from build123d import *

# Parameters (mm, degrees)
CROQUIS1_W              = 195
CROQUIS1_H              = 38
CROQUIS1_R              = 1.625
SALIENTE_EXTRUIR1_DEPTH = 3
SALIENTE_EXTRUIR2_START = -20
SALIENTE_EXTRUIR2_DEPTH = 16.5
CROQUIS3_W              = 10.5
CROQUIS3_H              = 7
CORTAR_EXTRUIR1_DEPTH   = 31.243984
SALIENTE_EXTRUIR3_START = -20
SALIENTE_EXTRUIR3_DEPTH = 16.5
CROQUIS5_W              = 10.5
CROQUIS5_H              = 7
CORTAR_EXTRUIR2_DEPTH   = 31.243984
SALIENTE_EXTRUIR4_START = -120
SALIENTE_EXTRUIR4_DEPTH = 45
CROQUIS7_R              = 8.25
CORTAR_EXTRUIR3_DEPTH   = 31.243984
CROQUIS8_W              = 195
CROQUIS8_H              = 3
SALIENTE_EXTRUIR5_DEPTH = 5
CORTAR_EXTRUIR4_REACH   = 122
CROQUIS10_W             = 55.675323807
CROQUIS10_H             = 32.604384831
SALIENTE_EXTRUIR7_DEPTH = 3


with BuildPart() as part:
    # Croquis1 → Saliente-Extruir1 (new body)
    with BuildSketch(Plane.XY):
        with Locations((0, 19)):
            Rectangle(CROQUIS1_W, CROQUIS1_H)
        with Locations((91.125, 15)):
            Circle(CROQUIS1_R, mode=Mode.SUBTRACT)
        with Locations((-91.125, 15)):
            Circle(CROQUIS1_R, mode=Mode.SUBTRACT)
    extrude(amount=SALIENTE_EXTRUIR1_DEPTH)

    # Croquis2 → Saliente-Extruir2 (add)
    with BuildSketch(Plane(origin=(97.5, 0, 0), x_dir=(0, 0, -1), z_dir=(1, 0, 0)).offset(SALIENTE_EXTRUIR2_START)):
        Polygon((3.429565646, 3.677896428), (15.185426147, 13.753887502), (0, 31.471028189), (0, 0.738403157), align=None)
    extrude(amount=-SALIENTE_EXTRUIR2_DEPTH)

    # Croquis3 → Cortar-Extruir1 (cut, through all)
    with BuildSketch(Plane(origin=(0, 0.425684191, 0.364855478), x_dir=(1, 0, 0), z_dir=(0, -0.759271307, -0.650774217))):
        with Locations((69.25, -11.980533736)):
            Rectangle(CROQUIS3_W, CROQUIS3_H)
    extrude(amount=-CORTAR_EXTRUIR1_DEPTH, mode=Mode.SUBTRACT)

    # Croquis4 → Saliente-Extruir3 (add)
    with BuildSketch(Plane.ZY.offset(97.5).offset(SALIENTE_EXTRUIR3_START)):
        Polygon((0, 0.738403157), (-15.185426147, 13.753887502), (0, 31.471028189), align=None)
    extrude(amount=-SALIENTE_EXTRUIR3_DEPTH)

    # Croquis5 → Cortar-Extruir2 (cut, through all)
    with BuildSketch(Plane(origin=(0, 0.425684191, 0.364855478), x_dir=(1, 0, 0), z_dir=(0, -0.759271307, -0.650774217))):
        with Locations((-69.25, -11.980533736)):
            Rectangle(CROQUIS5_W, CROQUIS5_H)
    extrude(amount=-CORTAR_EXTRUIR2_DEPTH, mode=Mode.SUBTRACT)

    # Croquis6 → Saliente-Extruir4 (add)
    with BuildSketch(Plane(origin=(97.5, 0, 0), x_dir=(0, 0, -1), z_dir=(1, 0, 0)).offset(SALIENTE_EXTRUIR4_START)):
        Polygon((0, 0.738403157), (15.185426147, 13.753887502), (0, 31.471028189), align=None)
    extrude(amount=SALIENTE_EXTRUIR4_DEPTH)

    # Croquis7 → Cortar-Extruir3 (cut, through all)
    with BuildSketch(Plane(origin=(0, 0.425684191, 0.364855478), x_dir=(1, 0, 0), z_dir=(0, -0.759271307, -0.650774217))):
        with Locations((-12.92, -10.480533736)):
            Circle(CROQUIS7_R)
        with Locations((12.93, -10.480533736)):
            Circle(CROQUIS7_R)
    extrude(amount=-CORTAR_EXTRUIR3_DEPTH, mode=Mode.SUBTRACT)

    # Croquis8 → Saliente-Extruir5 (add)
    with BuildSketch(Plane.XZ):
        with Locations((0, 1.5)):
            Rectangle(CROQUIS8_W, CROQUIS8_H)
    extrude(amount=SALIENTE_EXTRUIR5_DEPTH)

    # Croquis9 → Cortar-Extruir4 (cut, up to next)
    with BuildSketch(Plane.ZY.offset(22.5), mode=Mode.PRIVATE) as cortar_extruir4_sk1:
        Polygon((0, 0.738403157), (-15.185426147, 13.753887502), (0, 31.471028189), align=None)
    cortar_extruir4_tool1 = extrude(cortar_extruir4_sk1.sketch, amount=-CORTAR_EXTRUIR4_REACH, mode=Mode.PRIVATE) & part.part
    add(cortar_extruir4_tool1.solids().sort_by_distance((-22.5, 15.321106, -5.061809))[0], mode=Mode.SUBTRACT)

    # Croquis10 → Saliente-Extruir7 (add)
    with BuildSketch(Plane.XY.offset(3)):
        with Locations((-1.24159067, 18.458583135)):
            Rectangle(CROQUIS10_W, CROQUIS10_H)
    extrude(amount=-SALIENTE_EXTRUIR7_DEPTH)


solid = part.part
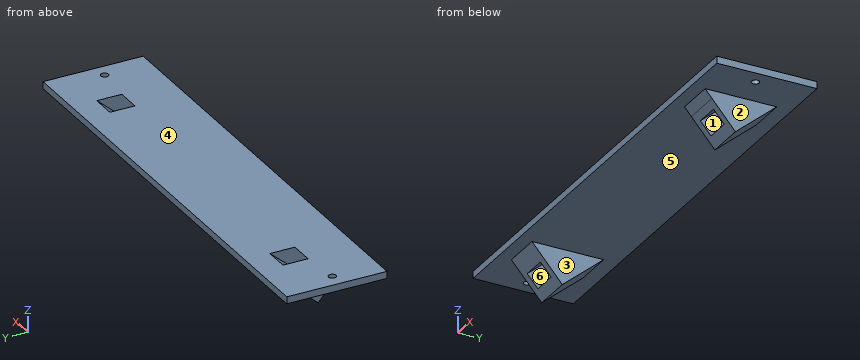
Geometry check sheet. Reference: the model listing, model coordinates, mm. Face numbers are marked on the shaded views. A direction names the side the tool comes from. Round coordinates to 2 decimals unless told otherwise and drop trailing zeros. Write each loop counter-clockwise with the first axis right and the second up, starting at its lowest first coordinate (ties: lowest second). Pieces come first, ordered by that corner, then holes. Notation, with made-up numbers: (3, -21) -> (56, -21) arc R22 cw to (56, -4) -> close; hole circle Ø11 at (17.25, 6). An arc over 180 degrees is marked (long way). One line per item, written item: value. Start each with the question number.
(1) Go/stop test with flat-tipped pins: pin 1 Ø21.5 at (x, y) = (26.5, 17.5) entering from -Z; pin 2 Ø4.5 at (y, z) = (20.5, -1) entering from +X; pin 3 Ø3 at (x, y) = (-60.5, 24) entering from -Z; pin 4 Ø7.5 at (y, z) = (21, -9) entering from -X. Record where each tip stops, or that it passes through.
(2) Draft check along Z on the marked faces 4, 5 and 6. Enter one of: +Z half, -Z half, draft (parallel to the pull), parting line (faces both ways), or undercut.
(3) Cross-section at A-A, the plane x = -72. Record the cut outline in (y, z).
(4) Scan lines: line 1 (X direction, y = 19, z = -2.75); line 2 (Z direction, x = -36, y = 18); line 3 (Z direction, x = 69.5, y = 6). Record each from-to range of solid material in increasing order. Write a range as [from, to].
(5) Cross-section at C-C, the plane y = 22. Record the cut outline in (x, z), and give its area (3 significant figures).
(6) Access from +Z, -Z, +X, -X, +Y, -Y to the whole of each face (thin tool, end or side, straight path). Record for the marked faces 1, 2 and 3.
(7) Cross-section at B-B, the plane z = -8.5. Record the cut outline in (x, y).
Answer:
1. pin 1: z = 0
1. pin 2: x = 97.5
1. pin 3: z = -7.62
1. pin 4: x = -77.5
2. face 4: +Z half
2. face 5: -Z half
2. face 6: undercut
3. outline: (-5, 0) -> (0.74, 0) -> (5.94, -6.07) -> (16.53, 3) -> (-5, 3) -> close; (10.5, -11.39) -> (13.75, -15.19) -> (31.47, 0) -> (38, 0) -> (38, 3) -> (27.29, 3) -> close
4. line 1: [-77.5, -74.5], [-64, -61], [61, 64], [74.5, 77.5]
4. line 2: [0, 3]
4. line 3: [-6.03, 3]
5. outline: (-97.5, 0) -> (-77.5, 0) -> (-77.5, -8.12) -> (-61, -8.12) -> (-61, 0) -> (61, 0) -> (61, -8.12) -> (77.5, -8.12) -> (77.5, 0) -> (97.5, 0) -> (97.5, 3) -> (74.5, 3) -> (74.5, -1.53) -> (64, -1.53) -> (64, 3) -> (-64, 3) -> (-64, -1.53) -> (-74.5, -1.53) -> (-74.5, 3) -> (-97.5, 3) -> close
5. area: 758 mm²
6. face 1: none
6. face 2: -Z, +X, +Y, -Y
6. face 3: -Z, +Y, -Y
7. outline: (-77.5, 8.02) -> (-74.5, 8.02) -> (-74.5, 13.87) -> (-64, 13.87) -> (-64, 8.02) -> (-61, 8.02) -> (-61, 21.55) -> (-77.5, 21.55) -> close; (61, 8.02) -> (64, 8.02) -> (64, 13.87) -> (74.5, 13.87) -> (74.5, 8.02) -> (77.5, 8.02) -> (77.5, 21.55) -> (61, 21.55) -> close
